Part model, mm, in its own coordinate system. Face numbers are marked on the shaded views. A direction names the side the tool comes from. Round coordinates to 2 decimals unless told otherwise and drop trailing zeros. Write each loop counter-clockwise with the first axis right and the second up, starting at its lowest first coordinate (ties: lowest second). Pieces come first, ordered by that corner, then holes. Notation, with made-up numbers: (-16, 85.25) -> (3, 85.25) arc R19 ccw to (3, 100.25) -> close; hole circle Ø10 at (-18, 15). An arc over 180 degrees is marked (long way). Use CSV: the item, a comma, the result in double quotes. Start each with the question number.
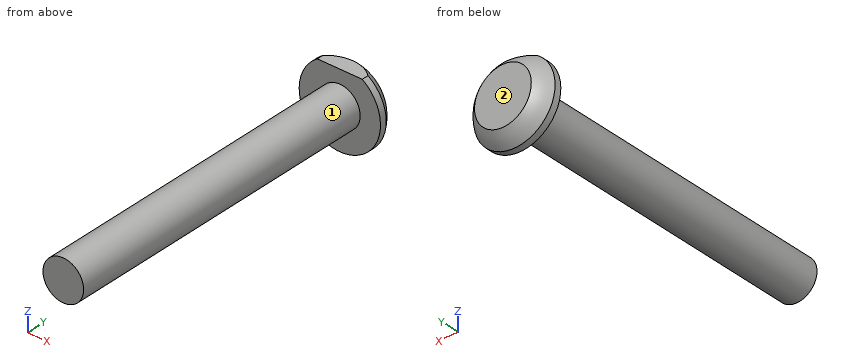
```python
from build123d import *

# Parameters (mm, degrees)
F0_R          = 4.7625
F1_DEPTH      = 76.2
F5_DEPTH      = 25.4
F5_DEPTH_BACK = 25.4
F7_DEPTH      = 25.4


with BuildPart() as f1:
    # F0 (on Front) → F1 (new body)
    with BuildSketch(Plane.XZ):
        Circle(F0_R)
    extrude(amount=F1_DEPTH)

    # F2 (on Right) → F3 (revolve)
    with BuildSketch(Plane.YZ):
        with BuildLine():
            Line((0, 9.525), (0, 0))
            Line((0, 0), (6.9723, 0))
            ThreePointArc((6.9723, 0), (5.5317575144, 5.4718273081), (1.5836126498, 9.525))
            Line((1.5836126498, 9.525), (0, 9.525))
        make_face()
    revolve(axis=Axis((0, 3.48615, 0), (0, 1, 0)))

    # F4 (on Right) → F5 (cut, two sides)
    with BuildSketch(Plane.YZ) as f5_sk:
        Polygon((4.7625, 7.9903732985), (4.7625, 0), (4.7625, -11.3777695224), (8.8222939521, -11.3777695224), (8.8222939521, 7.9903732985), align=None)
    extrude(amount=-F5_DEPTH, mode=Mode.SUBTRACT)
    extrude(f5_sk.sketch, amount=F5_DEPTH_BACK, mode=Mode.SUBTRACT)

    # F6 (on Front) → F7 (cut)
    with BuildSketch(Plane.XZ):
        Polygon((-8.7503455579, 7.9375), (0, 7.9375), (10.3095453233, 7.9375), (10.3095453233, 11.5658193827), (-8.7503455579, 11.5658193827), align=None)
    extrude(amount=-F7_DEPTH, mode=Mode.SUBTRACT)


solid = f1.part
```
1. Band-saw the part on D-D (z = 5.75). List the corners of the cut face in (x, y).
2. Band-saw the part on C-C (y = -55.5). List the corners of the cut face in (x, z) (1 decimal).
3. Drill centre lines: line 1 along Y through (x, z) = (0.25, 7.25); line 2 along X through (y, z) = (-8, 0.25); line 3 along Y through (x, z) = (0.5, -5.5). Where is each one in solid material? Low to high. Write a range as [from, to].
4. Band-saw the part on B-B (x = 0). List the corners of the cut face in (y, z) (1 decimal), then the cut area to 3 significant figures.
5. Flat gauge pins, fed straight in: pin 1 (1.5 mm diameter, centred on y = -20, z = 3.5, fed in from +X); pin 2 (10 mm diameter, centred on x = -1.5, y = -44, fed in from -Z); pin 3 (1 mm diameter, centred on x = 4, y = -59, fed in from -Z). Where does each tip first touch, or does it go through?
6. Which spindle directions (+Z, -Z, +X, -X, +Y, -Y) get a long thin tool onto all of the face, cutting with end or side? Do the marked faces 1 and 2. Say none if no direction does.
7. Band-saw the part on A-A (z = 0). List the corners of the cut face in (x, y) (1 decimal).
Answers below:
1,outline,"(-7.59, 0) -> (7.59, 0) -> (7.59, 1.58) arc R9.51 ccw to (3.34, 4.76) -> (-3.34, 4.76) arc R9.51 ccw to (-7.59, 1.58) -> close"
2,outline,"circle Ø9.5 at (0, 0)"
3,line 1,"y = [0, 4.28]"
3,line 2,"x = [-4.76, 4.76]"
3,line 3,"y = [0, 4.76]"
4,outline,"(-76.2, -4.8) -> (0, -4.8) -> (0, -9.5) -> (1.6, -9.5) arc R11.1 ccw to (4.8, -6.7) -> (4.8, 6.7) arc R11.1 ccw to (3.6, 7.9) -> (0, 7.9) -> (0, 4.8) -> (-76.2, 4.8) -> close"
4,area,"804 mm^2"
5,pin 1,"stops at x = 3.89"
5,pin 2,"stops at z = -4.76"
5,pin 3,"stops at z = -3.23"
6,face 1,"-Y"
6,face 2,"+Z, -Z, +X, -X, +Y"
7,outline,"(-9.5, 0) -> (-4.8, 0) -> (-4.8, -76.2) -> (4.8, -76.2) -> (4.8, 0) -> (9.5, 0) -> (9.5, 1.6) arc R11.1 ccw to (6.7, 4.8) -> (-6.7, 4.8) arc R11.1 ccw to (-9.5, 1.6) -> close"
